For this review, take the finished solid that the model builds, in its own axes (mm). Face numbers are marked on the shaded views. A direction names the side the tool comes from. Round coordinates to 2 decimals unless told otherwise and drop trailing zeros. Write each loop counter-clockwise with the first axis right and the second up, starting at its lowest first coordinate (ties: lowest second). Pieces come first, ordered by that corner, then holes. Notation, with made-up numbers: (53.5, -9) - (82.5, -9) arc R19 cw to (82.5, 18) - close; hole circle Ø3 at (71, 81.5). An arc over 180 degrees is marked (long way). Answer in a Markdown table with one row per item. Add a question column.
from build123d import *

# Parameters (mm, degrees)
F0_W     = 127
F0_H     = 76.2
F1_DEPTH = 94.996
F3_DEPTH = 25.4
F4_DEPTH = 115.824
F5_DEPTH = 110.998
F6_R     = 11.8361581928
F7_DEPTH = 300.736
F8_R     = 12.4713083384
F9_DEPTH = 188.468


with BuildPart() as f1:
    # F0 (on Front) → F1 (new body)
    with BuildSketch(Plane.XZ):
        with Locations((2.9599239826, 4.2708883941)):
            Rectangle(F0_W, F0_H)
    extrude(amount=F1_DEPTH)

    # F2 (on face) → F3 (join)
    with BuildSketch(Plane.XZ.offset(94.996)):
        with BuildLine():
            Line((26.9120044817, 42.3708883941), (21.8338499293, 42.3708883941))
            ThreePointArc((21.8338499293, 42.3708883941), (2.9599239826, 23.4969624475), (-15.914001964, 42.3708883941))
            Line((-15.914001964, 42.3708883941), (-20.9921565165, 42.3708883941))
            ThreePointArc((-20.9921565165, 42.3708883941), (2.9599239826, 18.418807895), (26.9120044817, 42.3708883941))
        make_face()
    extrude(amount=F3_DEPTH)

    # F4 (cut): a face of the model
    f4_faces = [f1.faces().sort_by_distance(p)[0] for p in [
        (2.9599239826, -94.996, 34.3605454342),
    ]]
    extrude(f4_faces, amount=-F4_DEPTH, mode=Mode.SUBTRACT)

    # F2 (on face) → F5 (join)
    with BuildSketch(Plane.XZ.offset(94.996)):
        with BuildLine():
            Line((26.9120044817, 42.3708883941), (21.8338499293, 42.3708883941))
            ThreePointArc((21.8338499293, 42.3708883941), (2.9599239826, 23.4969624475), (-15.914001964, 42.3708883941))
            Line((-15.914001964, 42.3708883941), (-20.9921565165, 42.3708883941))
            ThreePointArc((-20.9921565165, 42.3708883941), (2.9599239826, 18.418807895), (26.9120044817, 42.3708883941))
        make_face()
    extrude(amount=-F5_DEPTH)

    # F6 (on face) → F7 (cut)
    with BuildSketch(Plane.XY.offset(42.3708883941)):
        with Locations((-44.6284934878, -52.3529723287)):
            Circle(F6_R)
    extrude(amount=-F7_DEPTH, mode=Mode.SUBTRACT)

    # F8 (on face) → F9 (cut)
    with BuildSketch(Plane.XY.offset(42.3708883941)):
        with Locations((38.2470600307, -48.7860329449)):
            Circle(F8_R)
    extrude(amount=-F9_DEPTH, mode=Mode.SUBTRACT)


solid = f1.part
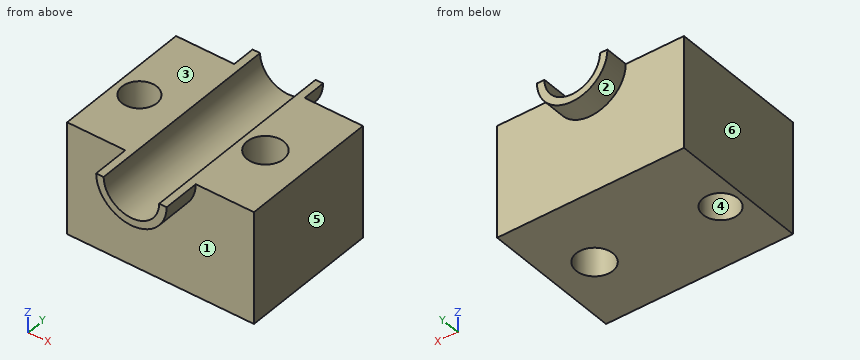
Q1. Tool access review of the marked faces 1, 2 and 3: name each direction out of +Z, -Z, +X, -X, +Y, -Y from which nothing blocks a thin tool from reaching the whole face with its end or side.
Q2. Insertion check: pin 1 Ø4 at (x, z) = (27.5, 18.5) entering from +Y; pin 2 Ø23 at (x, z) = (-22, 14) entering from -Y. Each pin has a flat end and moves straight along its axis. Give the tip position at first contact, or say it passes through.
Q3. Draft analysis for pull direction X (two halves, no side actions). For the marked faces 4, 5 and 6, state which applies: released by +X, released by -X, zero draft, split by the parting line, or undercut.
Q4. Add section C-C on y = -91.5. State the section outline as (x, z) points, then the cut area to 3 significant figures.
Q5. Add section A-A on z = 36. State the section outline as (x, y) points, then the cut area to 3 significant figures.
Q6. To check wall thickness, follow probe 1 along X at (y, z) = (-54, 28); probe 2 along X at (y, z) = (-48, -4.5); probe 3 along Y at (x, z) = (-22.5, 5.5). State the ranges of each line that lie inside material, in increasing order.
Q7. Add section B-B on x = 42.5. State the section outline as (y, z) points.
Q8. Add section D-D on z = 20.5. State the section outline as (x, y) points.
Answer sheet:
| question | item | result |
|---|---|---|
| 1 | face 1 | -Z, -Y |
| 1 | face 2 | -Z, +Y |
| 1 | face 3 | +Z, +X, -X, +Y, -Y |
| 2 | pin 1 | stops at y = 0 |
| 2 | pin 2 | stops at y = -95 |
| 3 | face 4 | undercut |
| 3 | face 5 | released by +X |
| 3 | face 6 | released by -X |
| 4 | outline | (-60.54, -33.83) - (66.46, -33.83) - (66.46, 42.37) - (21.83, 42.37) arc R18.87 cw to (-15.91, 42.37) - (-60.54, 42.37) - close |
| 4 | area | 9,120 mm² |
| 5 | outline | (-60.54, -95) - (-20.13, -95) - (-20.13, -120.4) - (-14.81, -120.4) - (-14.81, 16) - (-20.13, 16) - (-20.13, 0) - (-60.54, 0) - close; (20.73, -120.4) - (26.05, -120.4) - (26.05, -95) - (66.46, -95) - (66.46, 0) - (26.05, 0) - (26.05, 16) - (20.73, 16) - close; hole circle Ø23.67 at (-44.63, -52.35); hole circle Ø24.94 at (38.25, -48.79) |
| 5 | area | 8,200 mm² |
| 6 | probe 1 | x = -60.54 to -56.35, -32.91 to -9.28, 15.2 to 26.92, 49.58 to 66.46 |
| 6 | probe 2 | x = -60.54 to -55.64, -33.62 to 25.8, 50.69 to 66.46 |
| 6 | probe 3 | y = -95 to 0 |
| 7 | outline | (-95, -33.83) - (-60.51, -33.83) - (-60.51, 42.37) - (-95, 42.37) - close; (-37.06, -33.83) - (0, -33.83) - (0, 42.37) - (-37.06, 42.37) - close |
| 8 | outline | (-60.54, -95) - (-6.81, -95) - (-6.81, -120.4) - (12.73, -120.4) - (12.73, -95) - (66.46, -95) - (66.46, 0) - (12.73, 0) - (12.73, 16) - (-6.81, 16) - (-6.81, 0) - (-60.54, 0) - close; hole circle Ø23.67 at (-44.63, -52.35); hole circle Ø24.94 at (38.25, -48.79) |
